Can you work these out from the model? Positions are in its coordinate system, mm. Give positions to 0.01 mm unless a question says otherwise; leave off trailing zeros. Write each loop counter-clockwise with the first axis right and the second up, starting at its lowest first coordinate (ties: lowest second). Pieces come first, ordered by that corner, then holes.
Autodesk Inventor part; units mm, degrees
ref_plane "YZ Plane" through (0, 0, 0) normal (1, 0, 0) x (0, 1, 0)
ref_plane "XZ Plane" through (0, 0, 0) normal (0, 1, 0) x (-1, 0, 0)
ref_plane "XY Plane" through (0, 0, 0) normal (0, 0, 1) x (1, 0, 0)
sketch "Sketch1" plane through (0, 0, 0) normal (0, 1, 0) x (-1, 0, 0)
  circle A0 centre (0, 0) radius 80.645
  dimension "d4" = 161.29
extrude "Extrusion1" add sketch "Sketch1" against normal blind 6.35
sketch "Sketch2" plane through (0, 0, 0) normal (0, 1, 0) x (1, 0, 0)
  arc A0 (0, -80.645) -> (0, 80.645) centre (0, 0) ccw
  circle A1 centre (0, 0) radius 80.645
  line L0 (0, 80.645) -> (0, -80.645)
extrude "Extrusion2" cut sketch "Sketch2" against normal through all contours L0 A0
sketch "Sketch5" plane through (0, 0, 0) normal (0, 1, 0) x (1, 0, 0)
  circle A0 centre (0, 0) radius 63.5 construction
  circle A1 centre (-63.5, 0) radius 3.3782
  circle A2 centre (-51.3726, -37.3244) radius 3.3782
  circle A3 centre (-19.6226, -60.3921) radius 3.3782
  circle A4 centre (19.6226, -60.3921) radius 3.3782
  circle A5 centre (51.3726, -37.3244) radius 3.3782
  circle A6 centre (63.5, 0) radius 3.3782
  circle A7 centre (51.3726, 37.3244) radius 3.3782
  circle A8 centre (19.6226, 60.3921) radius 3.3782
  circle A9 centre (-19.6226, 60.3921) radius 3.3782
  circle A10 centre (-51.3726, 37.3244) radius 3.3782
  dimension "d17" = 127
  dimension "d18" = 6.7564
  dimension "d21" = 360
extrude "Extrusion3" cut sketch "Sketch5" against normal through all contours A1 | A2 | A3 | A9 | A10
properties part number "SupportPlateForWaterHalf" material "PET Plastic"
1) Please list where these lines run through material, in increasing order: L1, parallel to X at y = -3.75, z = 0 (3 decimals); L2, parallel to X at y = -2.5, z = -53.5; L3, parallel to Z at x = -23.5, y = -3.25.
Values follow:
L1: x = -80.645 to -66.878, -60.122 to 0
L2: x = -60.34 to 0
L3: z = -77.15 to 77.15
2) For pin 1 Ø1 at (x, y) = (-70.5, -4.5) entering from -Z; pin 2 Ø2 at (y, z) = (-2, 10.5) entering from -X; pin 3 Ø1.5 at (x, y) = (-69.5, -1) entering from +Z, each with a flat end and sliding along its axis, tell me the tip position at first contact or that it passes through.
Values follow:
pin 1: stops at z = -40.05
pin 2: stops at x = -80.08
pin 3: stops at z = 42.16
3) Suppose I cut it at A-A on z = 0. Write out the boundary of the cut face in (x, y) (3 decimals), plus the area to 3 significant figures.
Values follow:
outline: (-80.645, -6.35) - (-66.878, -6.35) - (-66.878, 0) - (-80.645, 0) - close; (-60.122, -6.35) - (0, -6.35) - (0, 0) - (-60.122, 0) - close
area: 469 mm2
4) Suppose I cut it at D-D on z = 21.5. Write out the boundary of the cut face in (x, y).
Values follow:
outline: (-77.73, -6.35) - (0, -6.35) - (0, 0) - (-77.73, 0) - close
5) Suppose I cut it at C-C on y = -1.5. Write out the boundary of the cut face in (x, z) (3 decimals), plus the area to 3 significant figures.
Values follow:
outline: (0, -80.645) - (0, 80.645) arc R80.645 ccw to start; hole circle Ø6.756 at (-63.5, 0); hole circle Ø6.756 at (-51.373, -37.324); hole circle Ø6.756 at (-51.373, 37.324); hole circle Ø6.756 at (-19.623, -60.392); hole circle Ø6.756 at (-19.623, 60.392)
area: 10,000 mm2
6) Suppose I cut it at B-B on x = -63.5. Write out the boundary of the cut face in (y, z).
Values follow:
outline: (-6.35, -49.71) - (0, -49.71) - (0, -3.38) - (-6.35, -3.38) - close; (-6.35, 3.38) - (0, 3.38) - (0, 49.71) - (-6.35, 49.71) - close
7) If we mould it in two halves opening along Z, with no side actions, what happens to faces 1 (the face through (-80.626, -3.131, -1.773)), 2 (the face through (-31, -6.35, 1)), 3 (the face through (-18.064, -3.131, 63.389))? For each: +Z half, -Z half, draft (parallel to the pull), parting line (faces both ways), or undercut.
Values follow:
face 1: parting line
face 2: draft
face 3: undercut
